```python
from build123d import *

# Parameters (mm, degrees)
F0_W      = 90
F0_H      = 90
F0_R      = 2.5
F0_R_2    = 19
F1_DEPTH  = 7
F3_W      = 12
F3_H      = 12
F4_DEPTH  = 60
F6_R      = 4.1
F7_DEPTH  = 100
F8_DEPTH  = 25
F12_DEPTH = 12
F15_DEPTH = 12


with BuildPart() as f1:
    # F0 (on Top) → F1 (new body)
    with BuildSketch(Plane.XY):
        Rectangle(F0_W, F0_H)
        with Locations((-23.55, -23.55)):
            Circle(F0_R, mode=Mode.SUBTRACT)
        with Locations((23.55, -23.55)):
            Circle(F0_R, mode=Mode.SUBTRACT)
        with Locations((-23.55, 23.55)):
            Circle(F0_R, mode=Mode.SUBTRACT)
        Circle(F0_R_2, mode=Mode.SUBTRACT)
        with Locations((23.55, 23.55)):
            Circle(F0_R, mode=Mode.SUBTRACT)
    extrude(amount=F1_DEPTH)

    # F3 (on offset) → F4 (join)
    with BuildSketch(Plane.XY.offset(7)):
        with Locations((-39, 39)):
            Rectangle(F3_W, F3_H)
        with Locations((39, 39)):
            Rectangle(F3_W, F3_H)
        with Locations((39, -39)):
            Rectangle(F3_W, F3_H)
        with Locations((-39, -39)):
            Rectangle(F3_W, F3_H)
    extrude(amount=F4_DEPTH)

    # F6 (on offset) → F7 (cut)
    with BuildSketch(Plane.XZ.offset(45)):
        with Locations((-39, 59.5)):
            Circle(F6_R)
        with Locations((39, 59.5)):
            Circle(F6_R)
    extrude(amount=-F7_DEPTH, mode=Mode.SUBTRACT)

    # F0 (on Top) → F8 (cut)
    with BuildSketch(Plane.XY):
        Circle(F0_R_2)
        with Locations((-23.55, 23.55)):
            Circle(F0_R)
        with Locations((23.55, 23.55)):
            Circle(F0_R)
        with Locations((23.55, -23.55)):
            Circle(F0_R)
        with Locations((-23.55, -23.55)):
            Circle(F0_R)
    extrude(amount=-F8_DEPTH, mode=Mode.SUBTRACT)

    # F11 (on face) → F12 (join)
    with BuildSketch(Plane.YZ.offset(45)):
        Polygon((0, 43), (-33, 66.4730164111), (-33, 54.4730164111), (-8.4352175508, 37), align=None)
        Polygon((33, 66.4730164111), (0, 43), (8.4352175508, 37), (33, 54.4730164111), align=None)
        Polygon((33, 19.5269835889), (8.4352175508, 37), (0, 31), (33, 7.5269835889), align=None)
        Polygon((0, 31), (-8.4352175508, 37), (-33, 19.5269835889), (-33, 7.5269835889), align=None)
        Polygon((8.4352175508, 37), (0, 43), (-8.4352175508, 37), (0, 31), align=None)
    extrude(amount=-F12_DEPTH)

    # F14 (on offset) → F15 (join)
    with BuildSketch(Plane(origin=(-45, 0, 0), x_dir=(0, -1, 0), z_dir=(-1, 0, 0))):
        Polygon((0, 43), (-33, 66.4730164111), (-33, 54.4730164111), (-8.4352175508, 37), (-33, 19.5269835889), (-33, 7.5269835889), (0, 31), (33, 7.5269835889), (33, 19.5269835889), (8.4352175508, 37), (33, 54.4730164111), (33, 66.4730164111), align=None)
    extrude(amount=-F15_DEPTH)


solid = f1.part
```
Source: CAD feature listing. Evaluate the final solid. Frame: model axes, mm. A direction names the side the tool comes from. Coordinates: 2 decimals unless noted, no trailing zeros. Write each loop counter-clockwise with the first axis right and the second up, starting at its lowest first coordinate (ties: lowest second). Pieces come first, ordered by that corner, then holes. Notation, with made-up numbers: (89.25, -15.5) -> (106.25, -15.5) arc R18 cw to (106.25, -3.5) -> close; hole circle Ø4 at (3, -24). An arc over 180 degrees is marked (long way). Return JSON: item names as keys, results as strings. Group by question number.
1) Mould query, pull axis Z, two halves, no side actions, for faces 6 (the face through (-39.08, -20.89, 28.14)), 7 (the face through (39.08, 16.73, 54.9)), 8 (the face through (33, -1, 37)). Classes: +Z half, -Z half, draft (parallel to the pull), parting line (faces both ways), or undercut.
2) Set-up query: faces 1 (the face through (-1, 21, 0)), 2 (the face through (23.01, -25.99, 3.45)), 3 (the face through (39, -33, 60)), 4 (the face through (-39.08, -16.73, 54.9)), 5 (the face through (39, -33, 37)). Return all of +Z, -Z, +X, -X, +Y, -Y with unobstructed straight access to the full face (end or side cutting, diameter ignored); none if empty.
3) Ray query, line 1 along Y through (x, z) = (23.55, 2.5); line 2 along X through (y, z) = (38, 59); line 3 along X through (y, z) = (37, 13). Return the intervals inside material, ascending.
4) Section query C-C, the plane z = 59.5. State how many separate pieces and enclosed holes the cut face has, plus the area to 3 significant figures.
5) Section query A-A, the plane x = 0. Return loops of the section in (y, z), plus the area to 3 significant figures.
6) Contact query for a flat-ended pin moving along its axis: P1, Ø4, axis at x = 18.5, y = 29.5, coming from the +Z side. Output: stop coordinate, or through.
7) Section query D-D, the plane y = 28. Return loops of the section in (x, z).
8) Section query B-B, the plane x = 39. Return loops of the section in (y, z).
From the geometry:
{
 "1": {"face 6": "undercut", "face 7": "+Z half", "face 8": "draft"},
 "2": {"face 1": "-Z, +X, -X, +Y, -Y", "face 2": "+Z, -Z", "face 3": "-Y", "face 4": "+Z, +X, -X", "face 5": "+X, -X"},
 "3": {"line 1": "-45 to -26.05, -21.05 to 21.05, 26.05 to 45", "line 2": "-45 to -43.07, -34.93 to -33, 33 to 34.93, 43.07 to 45", "line 3": "-45 to -33, 33 to 45"},
 "4": {"separate pieces": "4", "enclosed holes": "0", "area": "653 mm²"},
 "5": {"outline": "(-45, 0) -> (-19, 0) -> (-19, 7) -> (-45, 7) -> close; (19, 0) -> (45, 0) -> (45, 7) -> (19, 7) -> close", "area": "364 mm²"},
 "6": {"P1": "z = 7"},
 "7": {"outline": "(-45, 0) -> (45, 0) -> (45, 7) -> (-45, 7) -> close; (-45, 11.08) -> (-33, 11.08) -> (-33, 23.08) -> (-45, 23.08) -> close; (-45, 50.92) -> (-33, 50.92) -> (-33, 62.92) -> (-45, 62.92) -> close; (33, 11.08) -> (45, 11.08) -> (45, 23.08) -> (33, 23.08) -> close; (33, 50.92) -> (45, 50.92) -> (45, 62.92) -> (33, 62.92) -> close"},
 "8": {"outline": "(-45, 0) -> (45, 0) -> (45, 55.4) -> (33, 55.4) -> (33, 63.6) -> (45, 63.6) -> (45, 67) -> (33, 67) -> (33, 66.47) -> (0, 43) -> (-33, 66.47) -> (-33, 67) -> (-45, 67) -> (-45, 63.6) -> (-33, 63.6) -> (-33, 55.4) -> (-45, 55.4) -> close; hole (-33, 7) -> (33, 7) -> (33, 7.53) -> (0, 31) -> (-33, 7.53) -> close; hole (-33, 19.53) -> (-8.44, 37) -> (-33, 54.47) -> close; hole (8.44, 37) -> (33, 19.53) -> (33, 54.47) -> close"}
}
